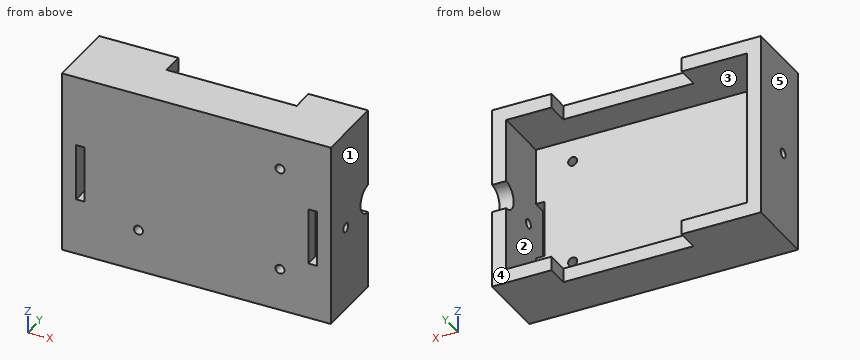
Autodesk Inventor part; units mm, degrees
ref_plane "YZ Plane" through (0, 0, 0) normal (1, 0, 0) x (0, 1, 0)
ref_plane "XZ Plane" through (0, 0, 0) normal (0, 1, 0) x (-1, 0, 0)
ref_plane "XY Plane" through (0, 0, 0) normal (0, 0, 1) x (1, 0, 0)
sketch "Sketch1" plane through (0, 0, 0) normal (0, 1, 0) x (-1, 0, 0)
  line L0 (0, 0) -> (95, 0)
  line L1 (95, 0) -> (95, 65)
  line L2 (95, 65) -> (0, 65)
  line L3 (0, 65) -> (0, 0)
  dimension "d0" = 95
  dimension "d1" = 65
extrude "Extrusion1" add sketch "Sketch1" along normal blind 25
sketch "Sketch2" plane through (0, 25, 0) normal (0, 1, 0) x (1, 0, 0)
  line L0 (-5, -5) -> (-90, -5)
  line L1 (-90, -5) -> (-90, -60)
  line L2 (-90, -60) -> (-5, -60)
  line L3 (-5, -60) -> (-5, -5)
extrude "Extrusion2" cut sketch "Sketch2" against normal blind 20
sketch "Sketch3" plane through (0, 25, 0) normal (0, 1, 0) x (1, 0, 0)
  line L0 (-5, -60) -> (-90, -60)
  line L1 (-95, -65) -> (0, -65)
  line L2 (-67, -65) -> (-67, -60)
  line L3 (-21, -60) -> (-21, -65)
  line L4 (-90, -5) -> (-5, -5)
  line L5 (0, 0) -> (-95, 0)
  line L6 (0, -65) -> (0, 0)
  line L7 (-67, -5) -> (-67, 0)
  line L8 (-21, -5) -> (-21, 0)
  line L9 (-67, 0) -> (-21, 0)
  line L10 (-21, -5) -> (-67, -5)
  dimension "d6" = 28
  dimension "d7" = 21
extrude "Extrusion4" cut sketch "Sketch3" against normal blind 8 contours L3 L1 L2 L0
extrude "Extrusion5" cut sketch "Sketch3" against normal blind 8 contours L8 L4 L7 L5
sketch "Sketch4" plane through (0, 0, 65) normal (1, 0, 0) x (0, 0, -1)
  line L0 (0, 25) -> (65, 25)
  circle A0 centre (32.5, 25) radius 5
  dimension "d14" = 10
extrude "Extrusion6" cut sketch "Sketch4" against normal blind 8
sketch "Sketch5" plane through (0, 5, 0) normal (0, 1, 0) x (1, 0, 0)
  line L0 (-90, -5) -> (-5, -5)
  line L1 (-90, -60) -> (-90, -5)
  line L2 (-90, -20) -> (-87, -20)
  line L3 (-87, -20) -> (-87, -40)
  line L4 (-87, -40) -> (-90, -40)
  line L5 (-90, -40) -> (-90, -20)
  point P0 (0, 0)
  dimension "d17" = 3
  dimension "d18" = 20
  dimension "d19" = 15
extrude "Extrusion7" cut sketch "Sketch5" against normal blind 8
sketch "Sketch6" plane through (0, 5, 0) normal (0, 1, 0) x (1, 0, 0)
  line L0 (-5, -5) -> (-5, -60)
  line L1 (-90, -20) -> (-90, -5)
  line L2 (-5, -20) -> (-8, -20)
  line L3 (-8, -20) -> (-8, -40)
  line L4 (-8, -40) -> (-5, -40)
  point P0 (0, 0)
  dimension "d22" = 3
  dimension "d23" = 20
extrude "Extrusion8" cut sketch "Sketch6" against normal blind 8
sketch "Sketch7" plane through (-95, 0, 0) normal (-1, 0, 0) x (0, 0, 1)
  line L0 (0, 0) -> (65, 0)
  line L1 (0, 0) -> (0, 25)
  circle A0 centre (30, 10) radius 1.625
  dimension "d26" = 3.25
  dimension "d27" = 10
  dimension "d28" = 30
hole "Hole1" at (-95, 10, 30) direction (1, 0, 0) diameter 3.25 end through all
sketch "Sketch8" plane through (0, 5, 0) normal (0, 1, 0) x (1, 0, 0)
  line L0 (-5, -5) -> (-5, -20)
  line L1 (-90, -5) -> (-5, -5)
  line L2 (-90, -20) -> (-90, -5)
  line L3 (-5, -60) -> (-90, -60)
  circle A0 centre (-68, -15) radius 1.6
  circle A1 centre (-18, -15) radius 1.6
  circle A2 centre (-18, -52) radius 1.6
  line L4 (-5, -40) -> (-5, -60)
  point P0 (0, 0)
  dimension "d36" = 3.2
  dimension "d39" = 3.2
  dimension "d50" = 22
  dimension "d51" = 10
  dimension "d52" = 10
  dimension "d53" = 13
  dimension "d54" = 13
  dimension "d55" = 8
hole "Hole2" at (-68, 5, 15) at (-18, 5, 15) at (-18, 5, 52) direction (0, -1, 0) diameter 3.2 end through all
properties part number "MAINCHAMBER"
Design review of the part built by this model. Coordinates are the model's own, in mm. Face numbers are marked on the shaded views. A direction names the side the tool comes from. Coordinates: 2 decimals unless noted, no trailing zeros. Order: outer loops, then holes, each group sorted by start corner. A loop starts at its lowest first (then second) coordinate and runs counter-clockwise, first axis right, second up. Notation, with made-up numbers: (65, 74) - (75, 74) arc R26 ccw to (75, 111) - close; hole circle Ø1 at (18.5, -29). An arc over 180 degrees is marked (long way). Put each result on its own line as item: value.
1) Insertion check: P1, Ø2.5, axis at y = 19.5, z = 2.5, coming from the +X side; P2, Ø16.5, axis at x = -61, z = 23.5, coming from the +Y side; P3, Ø1.5, axis at x = -34.5, z = 62.5, coming from the +Y side. Each pin has a flat end and moves straight along its axis. Give the tip position at first contact, or say it passes through.
Response values:
P1: stops at x = 0
P2: stops at y = 5
P3: stops at y = 17
2) The part is to be moulded in two halves that separate along X. For the marked faces 3, 4 and 5, say which applies: released by +X, released by -X, zero draft, split by the parting line, or undercut.
Response values:
face 3: undercut
face 4: zero draft
face 5: released by -X
3) Take a section at A-A, the plane x = -68. Give the boundary of the cut face in (y, z).
Response values:
outline: (0, 0) - (25, 0) - (25, 5) - (5, 5) - (5, 13.4) - (0, 13.4) - close; (0, 16.6) - (5, 16.6) - (5, 60) - (25, 60) - (25, 65) - (0, 65) - close
4) Take a section at B-B, the plane z = 15. Give the boundary of the cut face in (x, y), and give its area (3 significant figures).
Response values:
outline: (-95, 0) - (-69.6, 0) - (-69.6, 5) - (-90, 5) - (-90, 25) - (-95, 25) - close; (-66.4, 0) - (-19.6, 0) - (-19.6, 5) - (-66.4, 5) - close; (-16.4, 0) - (0, 0) - (0, 25) - (-5, 25) - (-5, 5) - (-16.4, 5) - close
area: 643 mm²
5) Take a section at C-C, the plane z = 52. Give the boundary of the cut face in (x, y), and give its area (3 significant figures).
Response values:
outline: (-95, 0) - (-19.6, 0) - (-19.6, 5) - (-90, 5) - (-90, 25) - (-95, 25) - close; (-16.4, 0) - (0, 0) - (0, 25) - (-5, 25) - (-5, 5) - (-16.4, 5) - close
area: 659 mm²
6) Tool access review of the marked faces 1 and 2: name each direction out of +Z, -Z, +X, -X, +Y, -Y from which nothing blocks a thin tool from reaching the whole face with its end or side.
Response values:
face 1: +Z, -Z, +X, +Y, -Y
face 2: +Y
7) Take a section at D-D, the plane x = -18. Give the boundary of the cut face in (y, z).
Response values:
outline: (0, 0) - (25, 0) - (25, 5) - (5, 5) - (5, 13.4) - (0, 13.4) - close; (0, 16.6) - (5, 16.6) - (5, 50.4) - (0, 50.4) - close; (0, 53.6) - (5, 53.6) - (5, 60) - (25, 60) - (25, 65) - (0, 65) - close
8) Wall thickness on L1, parallel to X at y = 1.1, z = 15; L2, parallel to Z at x = -24, y = 12.5; L3, parallel to X at y = 7, z = 48: over which ranges is each line inside the solid? List them lowest first. Write a range as from..to.
Response values:
L1: x = -95..-69.6, -66.4..-19.6, -16.4..0
L2: z = 0..5, 60..65
L3: x = -95..-90, -5..0
